Part model, mm, in its own coordinate system. A direction names the side the tool comes from. Give positions to 0.01 mm unless a question says otherwise; leave off trailing zeros. Write each loop counter-clockwise with the first axis right and the second up, starting at its lowest first coordinate (ties: lowest second). Pieces come first, ordered by that corner, then holes.
from build123d import *

# Parameters (mm, degrees)
BOSS_EXTRUDE1_DEPTH = 16
SKETCH2_W           = 3.5
SKETCH2_H           = 8
CUT_EXTRUDE1_DEPTH  = 69.492700341
CUT_EXTRUDE2_REACH  = 70.493
SKETCH3_R           = 2.1
FILLET1_R           = 2
SKETCH4_R           = 9
CUT_EXTRUDE3_DEPTH  = 12.5
SKETCH5_R           = 2
CUT_EXTRUDE4_DEPTH  = 71.008928002
FILLET2_R           = 4


with BuildPart() as part:
    # Sketch1 → Boss-Extrude1 (new body)
    with BuildSketch(Plane.XY):
        Polygon((0, 0), (-47, 0), (-47, 6), (-65, 6), (-65, 2), (-50, 2), (-50, -10.5), (-65, -10.5), (-65, -14.5), (-47, -14.5), (-47, -8.5), (0, -8.5), align=None)
    extrude(amount=BOSS_EXTRUDE1_DEPTH)

    # Sketch2 → Cut-Extrude1 (cut, through all)
    with BuildSketch(Plane(origin=(0, 0, 0), x_dir=(1, 0, 0), z_dir=(0, 1, 0))):
        with Locations((-6.75, -8)):
            Rectangle(SKETCH2_W, SKETCH2_H)
        with BuildLine():
            Line((-25.5, -10.25), (-10.5, -10.25))
            Line((-10.5, -10.25), (-10.5, -5.75))
            Line((-10.5, -5.75), (-25.5, -5.75))
            ThreePointArc((-25.5, -5.75), (-27.750000403, -8), (-25.5, -10.25))
        make_face()
    extrude(amount=-CUT_EXTRUDE1_DEPTH, mode=Mode.SUBTRACT)

    # Cut-Extrude2: up to this face of the body (flat: up to its plane)
    cut_extrude2_end = Plane(part.part.faces().sort_by_distance((-10.5, -4.25, 8))[0])
    # Sketch3 → Cut-Extrude2 (cut, up to the picked face)
    with BuildSketch(Plane(origin=(0, 0, 0), x_dir=(0, 0, -1), z_dir=(1, 0, 0)), mode=Mode.PRIVATE) as cut_extrude2_sk1:
        with Locations(Location((-8, -4.25, 0), (0, 0, 90))):
            Circle(SKETCH3_R)
    cut_extrude2_tool1 = split(extrude(cut_extrude2_sk1.sketch, amount=-CUT_EXTRUDE2_REACH, mode=Mode.PRIVATE), bisect_by=cut_extrude2_end, keep=Keep.BOTH, mode=Mode.PRIVATE)
    add(cut_extrude2_tool1.solids().sort_by(Axis((0, -4.25, 8), (-1, 0, 0)))[0], mode=Mode.SUBTRACT)

    # Fillet1
    fillet1_edges = [part.edges().sort_by_distance(p)[0] for p in [
        (-47, -8.5, 8),
        (-47, -14.5, 8),
        (-47, 6, 8),
        (-47, 0, 8),
    ]]
    fillet(fillet1_edges, radius=FILLET1_R)

    # Sketch4 → Cut-Extrude3 (cut)
    with BuildSketch(Plane(origin=(0, -10.5, 0), x_dir=(1, 0, 0), z_dir=(0, 1, 0))):
        with Locations((-57, -8)):
            Circle(SKETCH4_R)
    extrude(amount=CUT_EXTRUDE3_DEPTH, mode=Mode.SUBTRACT)

    # Sketch5 → Cut-Extrude4 (cut, through all)
    with BuildSketch(Plane(origin=(0, 6, 0), x_dir=(1, 0, 0), z_dir=(0, 1, 0))):
        with Locations(Location((-56.5, -8, 0), (0, 0, 180))):
            Circle(SKETCH5_R)
    extrude(amount=-CUT_EXTRUDE4_DEPTH, mode=Mode.SUBTRACT)

    # Fillet2
    fillet2_edges = [part.edges().sort_by_distance(p)[0] for p in [
        (-65, -14.5, 8),
        (-65, 6, 8),
    ]]
    fillet(fillet2_edges, radius=FILLET2_R - 0.0001)  # a hair under: the kernel refuses the full size


solid = part.part
1) Saw through at B-B (y = -7). Write the cut outline in (x, z), and give its area (3 significant figures).
Check result:
outline: (-50, 0) - (0, 0) - (0, 16) - (-50, 16) - (-50, 13.66) arc R9 cw to (-50, 2.34) - close; hole (-25.5, 5.75) - (-10.5, 5.75) - (-10.5, 10.25) - (-25.5, 10.25) arc R2.25 ccw to start; hole (-8.5, 4) - (-5, 4) - (-5, 12) - (-8.5, 12) - close
area: 681 mm2
2) Saw through at C-C (z = 8). State how many separate pieces and enclosed holes the cut face has, and give its area (3 significant figures).
Check result:
separate pieces: 7
enclosed holes: 0
area: 311 mm2
3) Mould opens along Y. For faces 1 (the flat face through (-7, -4, 4)), 2 (the flat face through (-50, -4, 1)), 3 (the flat face through (-54, 6, 8)) say: +Y half, -Y half, draft (parallel to the pull), parting line (faces both ways), or undercut.
Check result:
face 1: draft
face 2: undercut
face 3: +Y half
4) Drill centre lines: L1, parallel to Z at x = -56.5, y = 4.45; L2, parallel to Y at x = -52, z = 11; L3, parallel to X at y = -1, z = 2. Where is each one in solid material? Low to high.
Check result:
L1: z = 0 to 6, 10 to 16
L2: y = -14.5 to -10.5, 2 to 6
L3: x = -50 to 0
5) 3-axis set-ups, long thin cutter, end or side, ignore diameter. For faces 4 (the flat face through (-18, -4, 5.75)), 5 (the cylindrical face through (-9.486, -4.523, 10.082)), 6 (the flat face through (-47, -12, 8)), 7 (the flat face through (-47, 3, 8)): which of +Z, -Z, +X, -X, +Y, -Y reach the whole face in a straight line?
Check result:
face 4: +Y, -Y
face 5: +X
face 6: +Z, -Z, +X, -Y
face 7: +Z, -Z, +X, +Y
6) Saw through at A-A (x = -60). Write the cut outline in (y, z), and give its area (3 significant figures).
Check result:
outline: (-14.5, 0) - (-10.5, 0) - (-10.5, 16) - (-14.5, 16) - close; (2, 0) - (6, 0) - (6, 16) - (2, 16) - close
area: 128 mm2
7) Flat gauge pins, fed straight in: P1, Ø0.6, axis at y = 3.5, z = 4, coming from the +X side; P2, Ø6.5, axis at y = -3, z = 9, coming from the -X side; P3, Ø1.9, axis at y = -6.5, z = 1, coming from the -X side. Where does each tip first touch, or does it go through?
Check result:
P1: stops at x = -47
P2: stops at x = -49.07
P3: stops at x = -50
